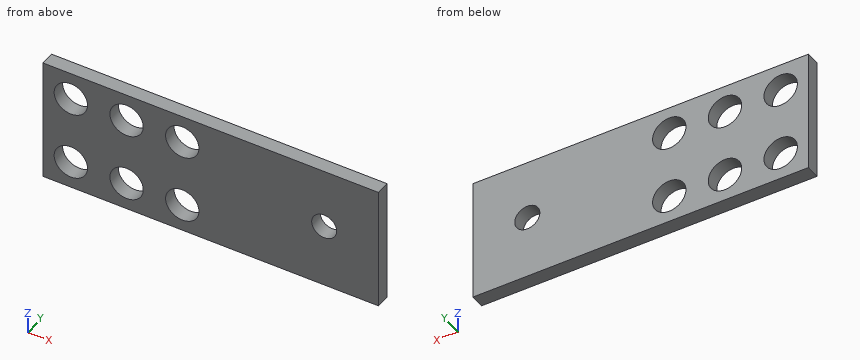
```python
from build123d import *

# Parameters (mm, degrees)
SKETCH1_W                  = 120.45107664
SKETCH1_H                  = 45
BOSS_EXTRUDE1_DEPTH        = 5
F_12_0_12_DIAMETER_HOLE1_D = 12
F_9_0_9_DIAMETER_HOLE1_D   = 9


with BuildPart() as part:
    # Sketch1 → Boss-Extrude1 (new body)
    with BuildSketch(Plane.XZ.offset(-74.218719002)):
        with Locations((-18.22553832, 310.029969029)):
            Rectangle(SKETCH1_W, SKETCH1_H)
    extrude(amount=BOSS_EXTRUDE1_DEPTH)

    # Ø12.0 (12) Diameter Hole1 (through all)
    with Locations(Plane(origin=(0, 74.218719002, 0), x_dir=(1, 0, 0), z_dir=(0, 1, 0))):
        with Locations((-68.45107664, -322.529969029), (-68.45107664, -297.529969029), (-48.45107664, -322.529969029), (-28.45107664, -322.529969029), (-48.45107664, -297.529969029), (-28.45107664, -297.529969029)):
            Hole(F_12_0_12_DIAMETER_HOLE1_D / 2)

    # Ø9.0 (9) Diameter Hole1 (through all)
    with Locations(Plane(origin=(0, 69.218719002, 0), x_dir=(-1, 0, 0), z_dir=(0, -1, 0))):
        with Locations((-22.5, -310.751020034)):
            Hole(F_9_0_9_DIAMETER_HOLE1_D / 2)


solid = part.part
```
Verification items for the finished model (mm, model axes). Give positions to 0.01 mm unless a question says otherwise; leave off trailing zeros. Order: outer loops, then holes, each group sorted by start corner. A loop starts at its lowest first (then second) coordinate and runs counter-clockwise, first axis right, second up. Notation, with made-up numbers: (82, 45) - (125, 45) arc R20 cw to (125, 73) - close; hole circle Ø3 at (-4.75, -34). An arc over 180 degrees is marked (long way). Answer as CSV lines item,"result". Start each with the question number.
Item 1: Section check A-A, the plane x = 22.5. Record the boundary of the cut face in (y, z), plus the area to 3 significant figures.
Item 2: Section check C-C, the plane y = 73.45. Record the boundary of the cut face in (x, z), plus the area to 3 significant figures.
Item 3: Section check B-B, the plane z = 312. Record the boundary of the cut face in (x, y).
Item 4: Section check D-D, the plane z = 299. Record the boundary of the cut face in (x, y), plus the area to 3 significant figures.
Item 5: Material ranges on L1, parallel to X at y = 69.6, z = 321; L2, parallel to X at y = 73.2, z = 298.5; L3, parallel to X at y = 72.75, z = 311, recorded low to high.
Filled in:
1,outline,"(69.22, 287.53) - (74.22, 287.53) - (74.22, 306.25) - (69.22, 306.25) - close; (69.22, 315.25) - (74.22, 315.25) - (74.22, 332.53) - (69.22, 332.53) - close"
1,area,"180 mm^2"
2,outline,"(-78.45, 287.53) - (42, 287.53) - (42, 332.53) - (-78.45, 332.53) - close; hole circle Ø12 at (-68.45, 297.53); hole circle Ø12 at (-68.45, 322.53); hole circle Ø12 at (-48.45, 297.53); hole circle Ø12 at (-48.45, 322.53); hole circle Ø12 at (-28.45, 297.53); hole circle Ø12 at (-28.45, 322.53); hole circle Ø9 at (22.5, 310.75)"
2,area,"4,680 mm^2"
3,outline,"(-78.45, 69.22) - (18.18, 69.22) - (18.18, 74.22) - (-78.45, 74.22) - close; (26.82, 69.22) - (42, 69.22) - (42, 74.22) - (26.82, 74.22) - close"
4,outline,"(-78.45, 69.22) - (-74.27, 69.22) - (-74.27, 74.22) - (-78.45, 74.22) - close; (-62.63, 69.22) - (-54.27, 69.22) - (-54.27, 74.22) - (-62.63, 74.22) - close; (-42.63, 69.22) - (-34.27, 69.22) - (-34.27, 74.22) - (-42.63, 74.22) - close; (-22.63, 69.22) - (42, 69.22) - (42, 74.22) - (-22.63, 74.22) - close"
4,area,"428 mm^2"
5,L1,"-78.45 to -74.25, -62.65 to -54.25, -42.65 to -34.25, -22.65 to 42"
5,L2,"-78.45 to -74.37, -62.53 to -54.37, -42.53 to -34.37, -22.53 to 42"
5,L3,"-78.45 to 18.01, 26.99 to 42"
